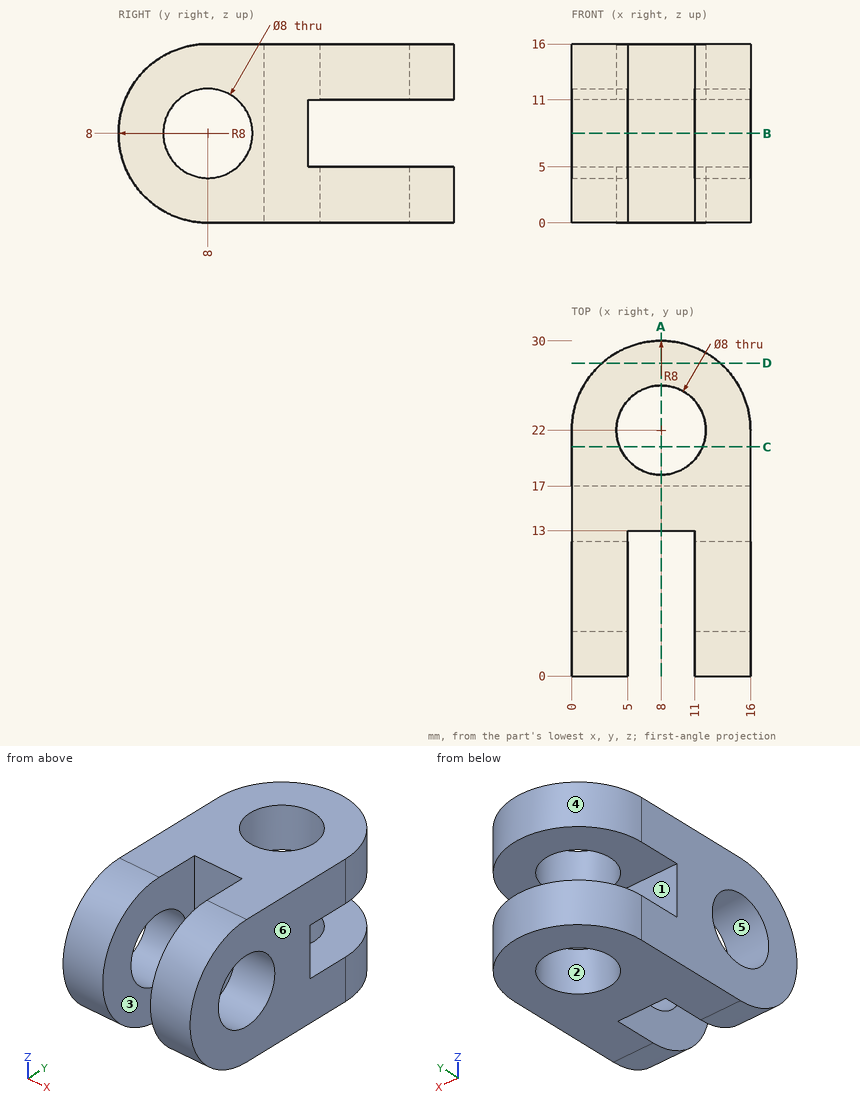
Part print with two shaded views. Sizes in mm from the minimum x, y, z corner. A direction names the side the tool comes from. Coordinates: 2 decimals unless noted, no trailing zeros. Loops run counter-clockwise (first coordinate to the right, second up) from the corner with the lowest first, then second, coordinate; pieces in that order, holes last. Notation, with made-up numbers: M 11.5,-31 L 47.5,-31 A7 ccw 47.5,-20 Z; hole C 77,-27 d4. An arc over 180 degrees is marked long. Use CSV: the item, a comma, the result in double quotes. Start each with the question number.
1. Band-saw the part on D-D, the plane y = 28. List the corners of the cut face in (x, z), then the cut area to 3 significant figures.
2. Probe probe 1 along Z at (x, y) = (3.95, 8); probe 2 along X at (y, z) = (11, 14.75). List the from-to ranges inside material, lowest first. Write a range as [from, to].
3. Flat gauge pins, fed straight in: pin 1 (1.5 mm diameter, centred on x = 5.5, z = 5.5, fed in from -Y); pin 2 (1.8 mm diameter, centred on x = 9.5, z = 7.5, fed in from +Y). Where does each tip first touch, or does it go through?
4. Two-plate mould, pull along Y, no slides. Class the marked faces 4, 5 and 6: pulls with the +Y half, pulls with the -Y half, needs draft (parallel to the pull), parting line crosses it, or undercut.
5. Band-saw the part on A-A, the plane x = 8. List the corners of the cut face in (y, z), then the cut area to 3 significant figures.
6. Band-saw the part on B-B, the plane z = 8. List the corners of the cut face in (x, y).
7. Band-saw the part on C-C, the plane y = 20.5. List the corners of the cut face in (x, z), then the cut area to 3 significant figures.
8. Tool access for the marked faces 1, 2 and 3: list every direction of +Z, -Z, +X, -X, +Y, -Y with a clear straight run to the whole face (end or side of a thin tool).
Entries:
1,outline,"M 2.71,0 L 13.29,0 L 13.29,5 L 2.71,5 Z; M 2.71,11 L 13.29,11 L 13.29,16 L 2.71,16 Z"
1,area,"106 mm2"
2,probe 1,"z = [0, 4], [12, 16]"
2,probe 2,"x = [0, 5], [11, 16]"
3,pin 1,"stops at y = 0.24"
3,pin 2,"stops at y = 17"
4,face 4,"pulls with the +Y half"
4,face 5,"undercut"
4,face 6,"needs draft"
5,outline,"M 13,0 L 18,0 L 18,5 L 17,5 L 17,11 L 18,11 L 18,16 L 13,16 Z; M 26,0 L 30,0 L 30,5 L 26,5 Z; M 26,11 L 30,11 L 30,16 L 26,16 Z"
5,area,"114 mm2"
6,outline,"M 0,0 L 5,0 L 5,4 L 0,4 Z; M 0,12 L 5,12 L 5,13 L 11,13 L 11,12 L 16,12 L 16,17 L 0,17 Z; M 11,0 L 16,0 L 16,4 L 11,4 Z"
7,outline,"M 0,0 L 4.29,0 L 4.29,5 L 0,5 Z; M 0,11 L 4.29,11 L 4.29,16 L 0,16 Z; M 11.71,0 L 16,0 L 16,5 L 11.71,5 Z; M 11.71,11 L 16,11 L 16,16 L 11.71,16 Z"
7,area,"85.8 mm2"
8,face 1,"+X, -X, +Y"
8,face 2,"+Z, -Z"
8,face 3,"+Z, -Z, -Y"
